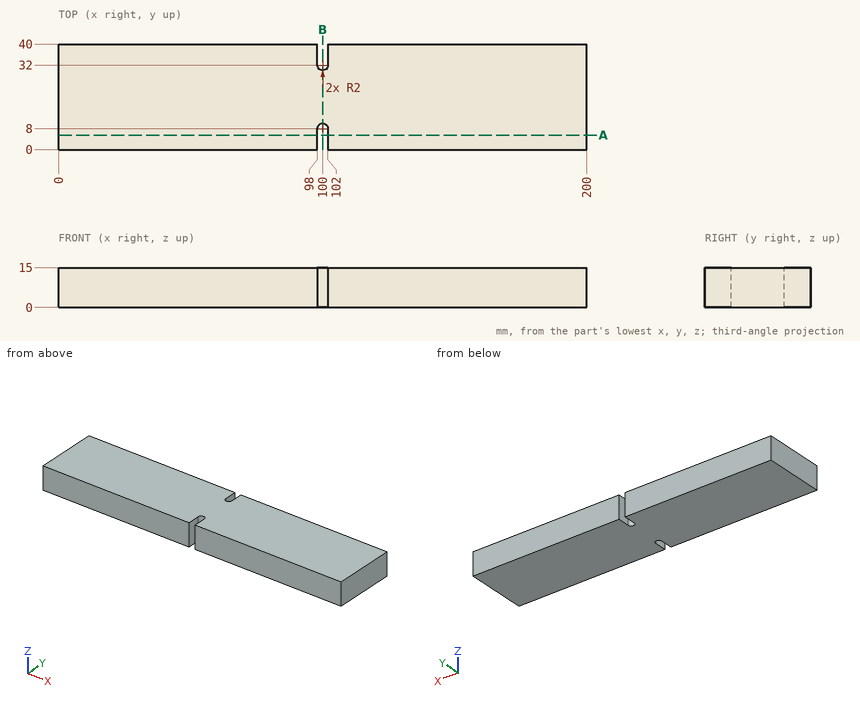
Print and shaded views of the part. All mm, measured from the part's lowest x, y and z. Coordinates: 2 decimals unless noted, no trailing zeros. Order: outer loops, then holes, each group sorted by start corner. A loop starts at its lowest first (then second) coordinate and runs counter-clockwise, first axis right, second up. Notation, with made-up numbers: (-3.5, 13) - (37.5, 13) arc R25 cw to (37.5, 25) - close; hole circle Ø2 at (68.25, 49). An arc over 180 degrees is marked (long way). Return JSON: item names as keys, results as strings. Group by question number.
Item 1: Drill centre lines: probe 1 along X at (y, z) = (3, 13.75); probe 2 along X at (y, z) = (8.5, 8.5). Where is each one in solid material? Low to high. Write a range as from..to.
Item 2: Pin check, flat tip, straight feed: pin 1 (6.5 mm diameter, centred on y = 36.5, z = 7.5, fed in from -X). Stop position of the tip, or through.
Item 3: Cut at A-A (y = 5.5). List the corners of the cut face in (x, z).
Item 4: Cut at B-B (x = 100). List the corners of the cut face in (y, z).
Check values:
{
 "1": {"probe 1": "x = 0..98, 102..200", "probe 2": "x = 0..98.06, 101.94..200"},
 "2": {"pin 1": "stops at x = 0"},
 "3": {"outline": "(0, 0) - (98, 0) - (98, 15) - (0, 15) - close; (102, 0) - (200, 0) - (200, 15) - (102, 15) - close"},
 "4": {"outline": "(10, 0) - (30, 0) - (30, 15) - (10, 15) - close"}
}
